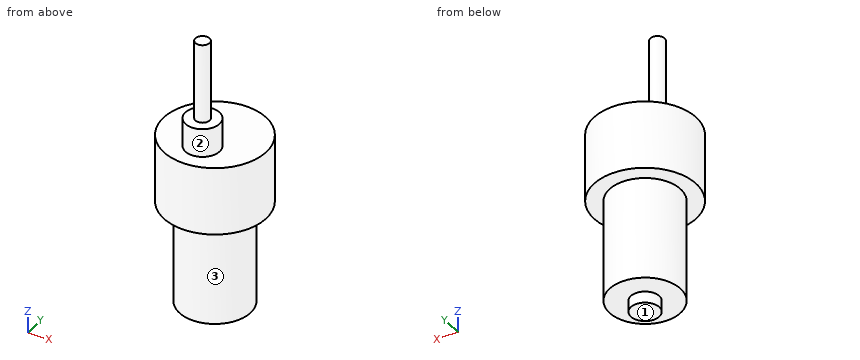
from build123d import *

# Parameters (mm, degrees)
SKETCH1_R           = 12.5
BOSS_EXTRUDE1_DEPTH = 36
SKETCH2_R           = 5
BOSS_EXTRUDE2_DEPTH = 4
SKETCH3_R           = 18
BOSS_EXTRUDE3_DEPTH = 24
SKETCH5_R           = 6
BOSS_EXTRUDE4_DEPTH = 10
SKETCH7_R           = 2.5
BOSS_EXTRUDE5_DEPTH = 28


with BuildPart() as part:
    # Sketch1 → Boss-Extrude1 (new body)
    with BuildSketch(Plane.XY):
        Circle(SKETCH1_R)
    extrude(amount=BOSS_EXTRUDE1_DEPTH)

    # Sketch2 → Boss-Extrude2 (add)
    with BuildSketch(Plane(origin=(0, 0, 0), x_dir=(-1, 0, 0), z_dir=(0, 0, -1))):
        Circle(SKETCH2_R)
    extrude(amount=BOSS_EXTRUDE2_DEPTH)

    # Sketch3 → Boss-Extrude3 (add)
    with BuildSketch(Plane.XY.offset(36)):
        Circle(SKETCH3_R)
    extrude(amount=BOSS_EXTRUDE3_DEPTH)

    # Sketch5 → Boss-Extrude4 (add)
    with BuildSketch(Plane.XY.offset(60)):
        with Locations((0, -7)):
            Circle(SKETCH5_R)
    extrude(amount=BOSS_EXTRUDE4_DEPTH)

    # Sketch7 → Boss-Extrude5 (add)
    with BuildSketch(Plane.XY.offset(70)):
        with Locations((0, -7)):
            Circle(SKETCH7_R)
    extrude(amount=BOSS_EXTRUDE5_DEPTH)


solid = part.part
Design review of the part built by this model. Coordinates are the model's own, in mm. Face numbers are marked on the shaded views. A direction names the side the tool comes from. Give positions to 0.01 mm unless a question says otherwise; leave off trailing zeros. Loops run counter-clockwise (first coordinate to the right, second up) from the corner with the lowest first, then second, coordinate; pieces in that order, holes last. Notation, with made-up numbers: (37, 84.5) -> (45, 84.5) arc R15 cw to (45, 109.5) -> close; hole circle Ø8 at (34, 42). An arc over 180 degrees is marked (long way). One line per question, with ' | ' between items. Start each with the question number.
(1) Insertion check: P1, Ø6, axis at x = 1, y = 9.5, coming from the -Z side; P2, Ø5, axis at x = 2, z = 32.5, coming from the +Y side; P3, Ø1, axis at x = -9, z = 17.5, coming from the +Y side. Each pin has a flat end and moves straight along its axis. Give the tip position at first contact, or say it passes through.
(2) For line 1 (Z direction, x = -5, y = -14); line 2 (Y direction, x = 0, z = 39.5); line 3 (Z direction, x = -2, y = 12), list the stretches that pass through material, from the lowest coordinate up.
(3) We need section B-B (y = 0). State the section outline as (x, z) points, and give its area (3 significant figures).
(4) We need section C-C (z = 16.5). State the section outline as (x, y) points, and give its area (3 significant figures).
(5) We need section D-D (y = -7). State the section outline as (x, z) points, and give its area (3 significant figures).
(6) For the marked faces 1, 2 and 3, list the 3-axis set-ups (+Z, -Z, +X, -X, +Y, -Y) from which the entire face can be reached by the end or side of a thin tool; tool diameter is ignored.
(7) We need section A-A (x = 0). State the section outline as (y, z) points.
The answers:
1) P1: stops at z = 0 | P2: stops at y = 12.5 | P3: stops at y = 9.17
2) line 1: z = 36 to 60 | line 2: y = -18 to 18 | line 3: z = 0 to 60
3) outline: (-18, 36) -> (-12.5, 36) -> (-12.5, 0) -> (-5, 0) -> (-5, -4) -> (5, -4) -> (5, 0) -> (12.5, 0) -> (12.5, 36) -> (18, 36) -> (18, 60) -> (-18, 60) -> close | area: 1,800 mm^2
4) outline: circle Ø25 at (0, 0) | area: 491 mm^2
5) outline: (-16.58, 36) -> (-10.36, 36) -> (-10.36, 0) -> (10.36, 0) -> (10.36, 36) -> (16.58, 36) -> (16.58, 60) -> (6, 60) -> (6, 70) -> (2.5, 70) -> (2.5, 98) -> (-2.5, 98) -> (-2.5, 70) -> (-6, 70) -> (-6, 60) -> (-16.58, 60) -> close | area: 1,800 mm^2
6) face 1: -Z, +X, -X, +Y, -Y | face 2: +Z | face 3: -Z
7) outline: (-18, 36) -> (-12.5, 36) -> (-12.5, 0) -> (-5, 0) -> (-5, -4) -> (5, -4) -> (5, 0) -> (12.5, 0) -> (12.5, 36) -> (18, 36) -> (18, 60) -> (-1, 60) -> (-1, 70) -> (-4.5, 70) -> (-4.5, 98) -> (-9.5, 98) -> (-9.5, 70) -> (-13, 70) -> (-13, 60) -> (-18, 60) -> close
